Source: CAD feature listing. Evaluate the final solid. Frame: model axes, mm. Face numbers are marked on the shaded views. A direction names the side the tool comes from. Give positions to 0.01 mm unless a question says otherwise; leave off trailing zeros. Write each loop counter-clockwise with the first axis right and the second up, starting at its lowest first coordinate (ties: lowest second). Pieces come first, ordered by that corner, then holes. Notation, with made-up numbers: M 22,1 L 50,1 A22 ccw 50,33 Z; hole C 52,-20.5 d10. An arc over 180 degrees is marked long. Answer as a JSON object with one key per item and string values. Group by question number.
```python
from build123d import *

# Parameters (mm, degrees)
BASE_EXTRUDE_DEPTH = 6.35
FILLET1_R          = 6.35
CUT_EXTRUDE1_DEPTH = 30.443738723


with BuildPart() as part:
    # Sketch1 → Base-Extrude (new, symmetric)
    with BuildSketch(Plane(origin=(0, 0, 0), x_dir=(1, 0, 0), z_dir=(0, 1, 0))):
        with BuildLine():
            Line((-28.575, 0), (-15.875, 0))
            ThreePointArc((-15.875, 0), (-13.282623356, -0.5532696), (-11.141989448, -2.116666667))
            ThreePointArc((-11.141989448, -2.116666667), (-10.071672494, -2.8983652), (-8.775484171, -3.175))
            Line((-8.775484171, -3.175), (8.775484171, -3.175))
            ThreePointArc((8.775484171, -3.175), (10.071672494, -2.8983652), (11.141989448, -2.116666667))
            ThreePointArc((11.141989448, -2.116666667), (13.282623356, -0.5532696), (15.875, 0))
            Line((15.875, 0), (28.575, 0))
            Line((28.575, 0), (28.575, -3.175))
            Line((28.575, -3.175), (15.875, -3.175))
            ThreePointArc((15.875, -3.175), (14.578811678, -3.4516348), (13.508494724, -4.233333333))
            ThreePointArc((13.508494724, -4.233333333), (11.367860816, -5.7967304), (8.775484171, -6.35))
            Line((8.775484171, -6.35), (-8.775484171, -6.35))
            ThreePointArc((-8.775484171, -6.35), (-11.367860816, -5.7967304), (-13.508494724, -4.233333333))
            ThreePointArc((-13.508494724, -4.233333333), (-14.578811678, -3.4516348), (-15.875, -3.175))
            Line((-15.875, -3.175), (-28.575, -3.175))
            Line((-28.575, -3.175), (-28.575, 0))
        make_face()
    extrude(amount=BASE_EXTRUDE_DEPTH, both=True)

    # Fillet1
    fillet1_edges = [part.edges().sort_by_distance(p)[0] for p in [
        (-28.575, 6.35, 1.5875),
        (28.575, 6.35, 1.5875),
        (28.575, -6.35, 1.5875),
        (-28.575, -6.35, 1.5875),
    ]]
    fillet(fillet1_edges, radius=FILLET1_R - 0.0001)  # a hair under: the kernel refuses the full size

    # Sketch2 → Cut-Extrude1 (cut, through all)
    with BuildSketch(Plane.XY.offset(3.175)):
        with BuildLine():
            Line((-22.895630041, -2.284864747), (-22.895630041, -2.908854561))
            Line((-22.895630041, -2.908854561), (-21.498676538, -2.908854561))
            Line((-21.498676538, -2.908854561), (-21.498676538, -2.267775516))
            ThreePointArc((-21.498676538, -2.267775516), (-22.254128161, 2.381071841), (-22.895630041, -2.284864747))
        make_face()
        with BuildLine():
            Line((21.498676538, -2.267775516), (21.498676538, -2.908854561))
            Line((21.498676538, -2.908854561), (22.895630041, -2.908854561))
            Line((22.895630041, -2.908854561), (22.895630041, -2.284864747))
            ThreePointArc((22.895630041, -2.284864747), (22.254128161, 2.381071841), (21.498676538, -2.267775516))
        make_face()
    extrude(amount=-CUT_EXTRUDE1_DEPTH, mode=Mode.SUBTRACT)


solid = part.part
```
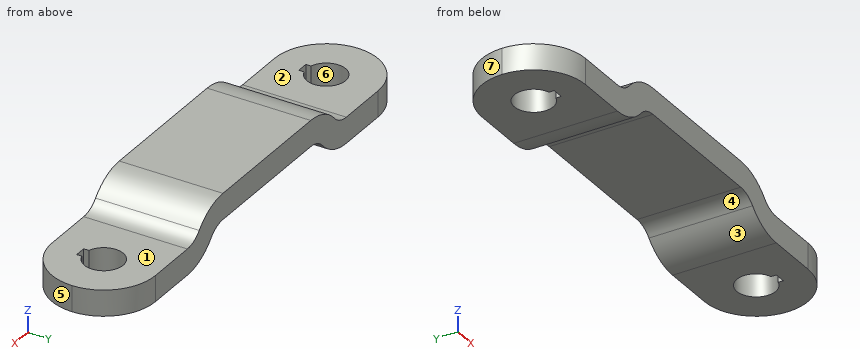
(1) Section A-A, the plane z = 0.5. State how many separate pieces and enclosed holes the cut face has, plus the area to 3 significant figures.
(2) Contact query for flat-ended pins moving along their axis: pin 1 Ø4 at (x, y) = (-1.5, -0.5) entering from -Z (3 decimals); pin 2 Ø0.7 at (y, z) = (-2.5, 1) entering from -X; pin 3 Ø1 at (y, z) = (1, 3.5) entering from -X. Output: stop coordinate, or through.
(3) Section B-B, the plane x = -24. Return loops of the section in (y, z) (3 decimals), plus the area to 3 significant figures.
(4) Ray query, L1, parallel to X at y = 0, z = 0.9 (3 decimals); L2, parallel to X at y = 0, z = 2.3 (3 decimals); L3, parallel to Z at x = -25, y = 4.25 (3 decimals). Return the intervals inside material, ascending. Write a range as [from, to].
(5) Pull-direction query (Y, two-part tool) for the marked faces 4, 5, 6 and 7; classes: pulls with the +Y half, pulls with the -Y half, needs draft (parallel to the pull), parting line crosses it, or undercut.
(6) Access query for the marked faces 1, 2 and 3. Directions: +Z, -Z, +X, -X, +Y, -Y. A direction counts if a zero-diameter tool reaches every point of the face in a straight line with its end or side. Return the directions, or none.
Reported:
{
 "1": {"separate pieces": "2", "enclosed holes": "2", "area": "314 mm2"},
 "2": {"pin 1": "stops at z = 3.175", "pin 2": "stops at x = -28.2", "pin 3": "stops at x = -28.54"},
 "3": {"outline": "M -6.097,0 L -1.587,0 L -1.587,3.175 L -6.097,3.175 Z; M 1.587,0 L 6.097,0 L 6.097,3.175 L 1.587,3.175 Z", "area": "28.6 mm2"},
 "4": {"L1": "x = [-28.575, -24.606], [-19.844, -12.616], [12.616, 19.844], [24.606, 28.575]", "L2": "x = [-28.575, -24.606], [-19.844, -10.964], [10.964, 19.844], [24.606, 28.575]", "L3": "z = [0, 3.175]"},
 "5": {"face 4": "needs draft", "face 5": "pulls with the -Y half", "face 6": "undercut", "face 7": "pulls with the +Y half"},
 "6": {"face 1": "+Z, +X, +Y, -Y", "face 2": "+Z, -X, +Y, -Y", "face 3": "-Z, +Y, -Y"}
}
